Autodesk Inventor part; units mm, degrees
ref_plane "YZ Plane" through (0, 0, 0) normal (1, 0, 0) x (0, 1, 0)
ref_plane "XZ Plane" through (0, 0, 0) normal (0, 1, 0) x (-1, 0, 0)
ref_plane "XY Plane" through (0, 0, 0) normal (0, 0, 1) x (1, 0, 0)
sketch "Skizze1" plane through (0, 0, 0) normal (0, 0, 1) x (1, 0, 0)
  line L0 (-56, 0) -> (-56, 90)
  line L1 (-56, 90) -> (-46, 90)
  line L2 (-46, 90) -> (21, 70.7881)
  line L3 (21, 70.7881) -> (21, 51)
  line L4 (21, 51) -> (51, 51)
  line L5 (51, 51) -> (51, 54)
  line L6 (51, 54) -> (56, 54)
  line L7 (56, 54) -> (56, 0)
  line L8 (-56, 0) -> (56, 0)
  point P0 (0, 0)
  point P1 (53.5, 54)
  point P2 (0, 0)
  dimension "d0" = 112
  dimension "d1" = 16
  dimension "d2" = 108
  dimension "d3" = 180
  dimension "d4" = 102
  dimension "d5" = 77
  dimension "d6" = 10
  dimension "d7" = 5
revolve "Umdrehung1" add sketch "Skizze1" angle 360 about axis through (-56, 0, 0) along (1, 0, 0)
fillet "Rundung1" radius 1.2 1 edges at (51, -51, 0)
fillet "Rundung2" radius 1.5 1 edges at (51, -54, 0)
fillet "Rundung3" radius 1.5 1 edges at (56, -54, 0)
sketch "Skizze2" plane through (21, 0, 0) normal (1, 0, 0) x (0, 0, -1)
  circle A0 centre (0, 0) radius 90
  line L0 (126, 0) -> (-126, 0)
  circle A1 centre (0, 0) radius 90
  circle A2 centre (0, 0) radius 70.7881
  arc A3 (-69.2826, -14.5216) -> (-69.2826, 14.5216) centre (-76, 0) ccw
  line L1 (-88.8207, 14.5216) -> (-69.2826, 14.5216)
  line L2 (-69.2826, -14.5216) -> (-88.8207, -14.5216)
  point P0 (0, 0)
  point P1 (-79.0517, 14.5216)
  point P2 (-79.0517, 14.5216)
  dimension "d16" = 16
  dimension "d54" = 76
extrude "Extrusion3" cut sketch "Skizze2" against normal blind 67 contours L1 A2 L0 A0 | A0 L0 A2 L2 | A3 L0 A2 | A2 L0 A3 picked at (-76.7377, 8.0985) picked at (-76.7377, -8.0985) picked at (-67.2736, 2.8267) picked at (-67.2736, -2.8267)
sketch "Skizze9" plane through (-46, 0, 0) normal (1, 0, 0) x (0, 0, -1)
  arc A0 (-69.2826, -14.5216) -> (-69.2826, 14.5216) centre (-76, 0) ccw
  point P0 (0, 0)
hole "Bohrung3" at (-46, 0, 76) direction (-1, 0, 0) diameter 8.5 end through all
pattern_circular "Runde Anordnung1" count 6 over 360 about axis through (-12.5, 0, 0) along (1, 0, 0) of "Extrusion3", "Bohrung3"
chamfer "Fasen1" distance 1 angle 45 1 edges at (-56, -90, 0)
chamfer "Fasen3" distance 3 angle 60 1 edges at (21, -51, 0) measured on face at (21, 19.1412, 59.8068)
sketch "Skizze11" plane through (-56, 0, 0) normal (-1, 0, 0) x (0, 0, 1)
  circle A0 centre (0, 0) radius 90
  point P0 (0, 0)
  point P1 (0, 0)
hole "Bohrung4" at (-56, 0, 0) direction (1, 0, 0) diameter 92 depth 79 counterbore diameter 98 counterbore depth 7
sketch "Skizze12" plane through (56, 0, 0) normal (1, 0, 0) x (0, 0, -1)
  circle A0 centre (0, 0) radius 54
  point P0 (0, 0)
hole "Bohrung5" at (56, 0, 0) direction (-1, 0, 0) diameter 93 depth 40
chamfer "Fasen4" distance 1 angle 60 1 edges at (-56, 0, -49) measured on face at (-56, 18.4136, -67.5369)
chamfer "Fasen5" distance 1.6 angle 60 1 edges at (-49, 0, -46) measured on face at (-49, 0, -46.8427)
fillet "Rundung6" radius 0.4 1 edges at (-49, 0, -49)
properties part number "bauteil_externe" material "Stahl, galvanisiert"
Build history of the part. All positions in model axes, mm. A direction names the side the tool comes from. Round coordinates to 2 decimals unless told otherwise and drop trailing zeros. Loops run counter-clockwise (first coordinate to the right, second up) from the corner with the lowest first, then second, coordinate; pieces in that order, holes last.
Item 1: Saw through at B-B (y = 0). State how many separate pieces and enclosed holes the cut face has, then the cut area to 3 significant figures.
Item 2: Saw through at A-A (x = -2). List the corners of the cut face in (y, z), then the cut area to 3 significant figures.
Item 3: Pin check, flat tips, straight feed: P1, Ø21.5, axis at x = -3.5, z = 82.5, coming from the -Y side; P2, Ø8, axis at x = 9.5, z = -3, coming from the -Y side; P3, Ø10, axis at x = -13.5, z = -78.5, coming from the -Y side. Stop position of each tip, or through.
Item 4: Drill centre lines: line 1 along Y through (x, z) = (-51, 0); line 2 along Z through (x, y) = (-11, 0); line 3 along Y through (x, z) = (-50, -38). Where is each one in solid material? Low to high.
Item 5: Two-plate mould, pull along Z, no slides. Class faces 1 (the face through (38.163, -11.056, -49.787)), 2 (the face through (-56, 38, -38)), 3 (the face through (-46, -61, 39)): released by +Z, released by -Z, zero draft, split by the parting line, or undercut.
Item 6: Which spindle directions (+Z, -Z, +X, -X, +Y, -Y) get a long thin tool onto all of the face, cutting with end or side? Do faces 4 (the face through (-26.92, 57.56, -50)), 5 (the face through (-51.8, -41.32, 26.34)), 6 (the face through (-27, 14.522, 75)), 7 (the face through (-51.07, 63.23, 34.63)), 8 (the face through (16, -45, 11)). Say none if no direction does.
Item 7: Saw through at C-C (x = 33.5). List the corners of the cut face in (y, z), then the cut area to 3 significant figures.
Worked answers:
1. separate pieces: 4
1. enclosed holes: 0
1. area: 2,890 mm2
2. outline: (-73.09, -25.43) - (-67.26, -22.07) arc R16 cw to (-52.74, -47.22) - (-58.56, -50.58) arc R77.38 ccw to (-14.52, -76.01) - (-14.52, -69.28) arc R16 cw to (14.52, -69.28) - (14.52, -76.01) arc R77.38 ccw to (58.56, -50.58) - (52.74, -47.22) arc R16 cw to (67.26, -22.07) - (73.09, -25.43) arc R77.38 ccw to (73.09, 25.43) - (67.26, 22.07) arc R16 cw to (52.74, 47.22) - (58.56, 50.58) arc R77.38 ccw to (14.52, 76.01) - (14.52, 69.28) arc R16 cw to (-14.52, 69.28) - (-14.52, 76.01) arc R77.38 ccw to (-58.56, 50.58) - (-52.74, 47.22) arc R16 cw to (-67.26, 22.07) - (-73.09, 25.43) arc R77.38 ccw to start; hole circle Ø92 at (0, 0)
2. area: 9,670 mm2
3. P1: stops at y = -31.31
3. P2: stops at y = -75.18
3. P3: stops at y = -33.81
4. line 1: y = -90 to -49, 49 to 90
4. line 2: z = -60 to -46, 46 to 60
4. line 3: y = -81.58 to -70.07, -61.57 to -30.94, 30.94 to 61.57, 70.07 to 81.58
5. face 1: split by the parting line
5. face 2: zero draft
5. face 3: undercut
6. face 4: +X, +Y
6. face 5: -X
6. face 6: +Z, +X
6. face 7: +X, -X
6. face 8: +X
7. outline: circle Ø102 at (0, 0); hole circle Ø93 at (0, 0)
7. area: 1,380 mm2
